from build123d import *

# Parameters (mm, degrees)
BOSS_EXTRUDE1_DEPTH      = 12.525
BOSS_EXTRUDE1_DEPTH_BACK = 12.525
SKETCH2_R                = 6
SKETCH2_R_2              = 3.5
CUT_EXTRUDE1_DEPTH       = 1
SKETCH3_R                = 1.6
CUT_EXTRUDE2_DEPTH       = 3
CHAMFER1_SIZE            = 2


with BuildPart() as part:
    # Sketch1 → Boss-Extrude1 (new, two sides: drawn at the far end of the back side and taken through both)
    with BuildSketch(Plane.XY.offset(-BOSS_EXTRUDE1_DEPTH_BACK)):
        with BuildLine():
            Line((-32.5, 12.5), (32.5, 12.5))
            ThreePointArc((32.5, 12.5), (45, 0), (32.5, -12.5))
            Line((32.5, -12.5), (-32.5, -12.5))
            ThreePointArc((-32.5, -12.5), (-45, 0), (-32.5, 12.5))
        make_face()
    extrude(amount=BOSS_EXTRUDE1_DEPTH + BOSS_EXTRUDE1_DEPTH_BACK)

    # Sketch2 → Cut-Extrude1 (cut)
    with BuildSketch(Plane.XY.offset(12.525)):
        with Locations((-32.5, 0)):
            Circle(SKETCH2_R)
        with Locations((-11.5, 0)):
            Circle(SKETCH2_R_2)
        with Locations((17.5, 0)):
            Circle(SKETCH2_R)
        with Locations((32.5, 0)):
            Circle(SKETCH2_R_2)
    extrude(amount=-CUT_EXTRUDE1_DEPTH, mode=Mode.SUBTRACT)

    # Sketch3 → Cut-Extrude2 (cut)
    with BuildSketch(Plane(origin=(0, 0, -12.525), x_dir=(-1, 0, 0), z_dir=(0, 0, -1))):
        with Locations((22.5, 0)):
            Circle(SKETCH3_R)
        with Locations((-22.5, 0)):
            Circle(SKETCH3_R)
    extrude(amount=-CUT_EXTRUDE2_DEPTH, mode=Mode.SUBTRACT)

    # Chamfer1
    chamfer1_edges = [part.edges().sort_by_distance(p)[0] for p in [
        (-45, 0, 12.525),
        (45, 0, -12.525),
        (0, -12.5, 12.525),
        (45, 0, 12.525),
        (0, 12.5, 12.525),
        (0, 12.5, -12.525),
        (-45, 0, -12.525),
        (0, -12.5, -12.525),
    ]]
    chamfer(chamfer1_edges, length=CHAMFER1_SIZE)


solid = part.part
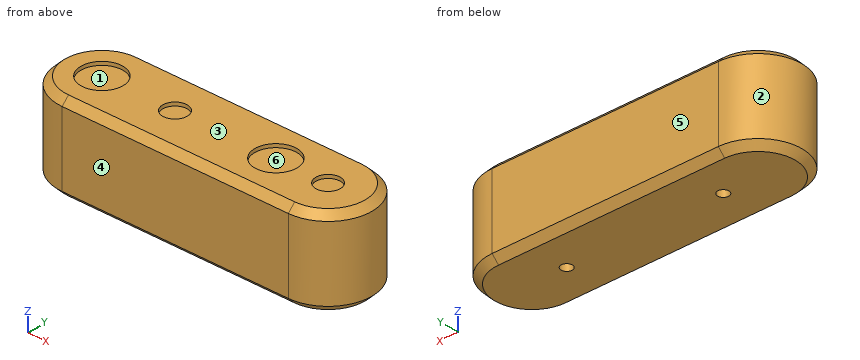
For this review, take the finished solid that the model builds, in its own axes (mm). Face numbers are marked on the shaded views. A direction names the side the tool comes from. Coordinates: 2 decimals unless noted, no trailing zeros. Order: outer loops, then holes, each group sorted by start corner. A loop starts at its lowest first (then second) coordinate and runs counter-clockwise, first axis right, second up. Notation, with made-up numbers: (74, -16) - (80, -16) arc R4 ccw to (80, -12) - close; hole circle Ø5 at (3.25, -38). An arc over 180 degrees is marked (long way). Use one line per item in the form item = value.
Q1. For the marked faces 5 and 6, list the 3-axis set-ups (+Z, -Z, +X, -X, +Y, -Y) from which the entire face can be reached by the end or side of a thin tool; tool diameter is ignored.
Checked values:
face_5 = +Z, -Z, +X, -X, +Y
face_6 = +Z
Q2. Consider section B-B (x = -11.5). Give the boundary of the cut face in (y, z) (3 decimals), then the cut area to 3 significant figures.
Checked values:
outline = (-12.5, -10.525) - (-10.5, -12.525) - (10.5, -12.525) - (12.5, -10.525) - (12.5, 10.525) - (10.5, 12.525) - (3.5, 12.525) - (3.5, 11.525) - (-3.5, 11.525) - (-3.5, 12.525) - (-10.5, 12.525) - (-12.5, 10.525) - close
area = 611 mm2
Q3. Consider section D-D (x = -30). Give the boundary of the cut face in (y, z) (3 decimals).
Checked values:
outline = (-12.5, -10.525) - (-10.5, -12.525) - (10.5, -12.525) - (12.5, -10.525) - (12.5, 10.525) - (10.5, 12.525) - (5.454, 12.525) - (5.454, 11.525) - (-5.454, 11.525) - (-5.454, 12.525) - (-10.5, 12.525) - (-12.5, 10.525) - close
Q4. For probe 1 along Y at (x, z) = (-22.5, -10.3); probe 2 along Y at (x, z) = (-32.5, 11.8) (3 decimals); probe 3 along Z at (x, y) = (-33, 2.75) (3 decimals), list the stretches that pass through material, from the lowest coordinate up. Write a range as from..to.
Checked values:
probe_1 = -12.5..-1.6, 1.6..12.5
probe_2 = -11.225..-6, 6..11.225
probe_3 = -12.525..11.525
Q5. For P1, Ø10, axis at y = 10, z = 1.5, coming from the -X side; P2, Ø6, axis at y = -3, z = 1.5, coming from the +X side; P3, Ø3.5, axis at x = 33.5, y = 0, coming from the +Z side (3 decimals); P4, Ø1.6, axis at x = -22.5, y = 0, coming from the -Z side (3 decimals), all flat-tipped, find the tip position at first contact; note any pin that passes through.
Checked values:
P1 = -43.96
P2 = 45
P3 = 11.525
P4 = -9.525
Q6. Consider section C-C (z = 5.25). Give the boundary of the cut face in (x, y).
Checked values:
outline = (-32.5, -12.5) - (32.5, -12.5) arc R12.5 ccw to (32.5, 12.5) - (-32.5, 12.5) arc R12.5 ccw to start
Q7. Draft analysis for pull direction Y (two halves, no side actions). For the marked faces 1, 2, 3 and 4, state which applies: +Y half, -Y half, draft (parallel to the pull), parting line (faces both ways), or undercut.
Checked values:
face_1 = undercut
face_2 = parting line
face_3 = draft
face_4 = -Y half
